Geometry: see drawing. Coordinates: mm, zero at the bounding-box minimum. A direction names the side the tool comes from. Give positions to 0.01 mm unless a question says otherwise; leave off trailing zeros. Loops run counter-clockwise (first coordinate to the right, second up) from the corner with the lowest first, then second, coordinate; pieces in that order, holes last. Notation, with made-up numbers: (30.25, -10) -> (49.25, -10) arc R33 ccw to (49.25, 18) -> close; hole circle Ø11 at (78, 16.5). An arc over 180 degrees is marked (long way). One line per question, with ' | ' between items.
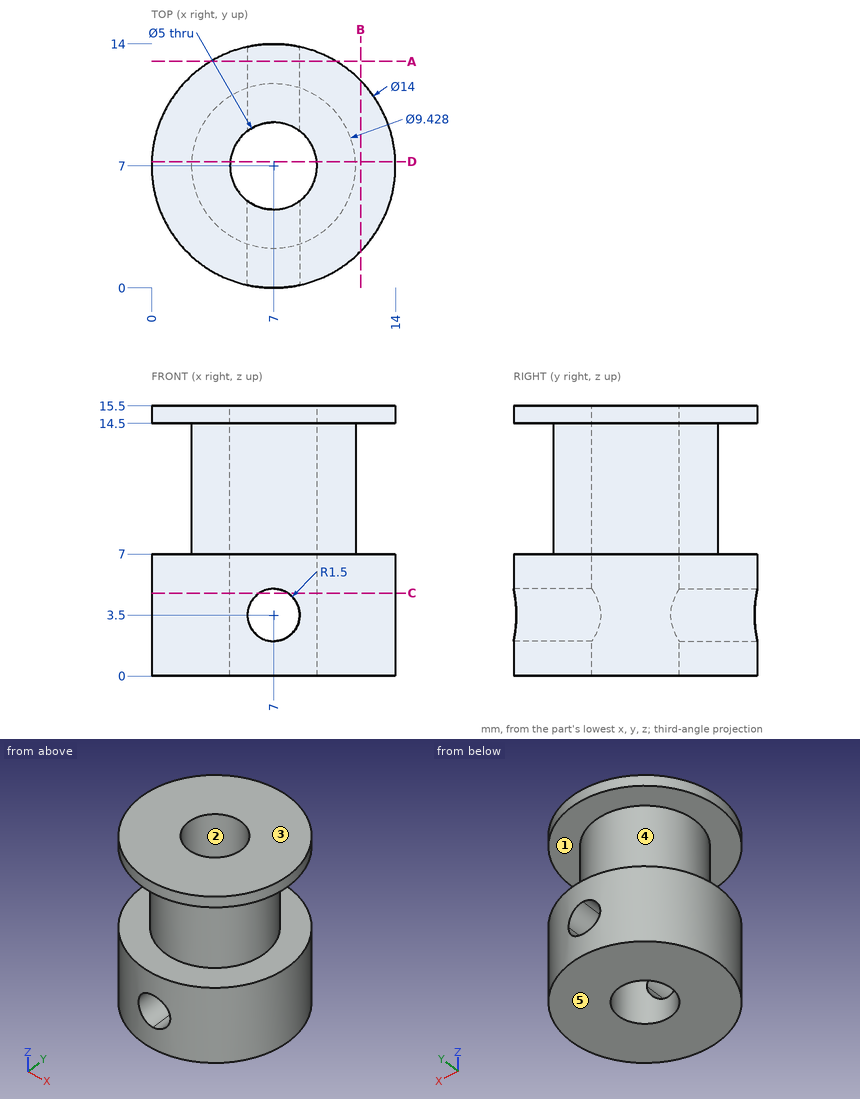
1. Reachability of the marked faces 1 and 2 from +Z, -Z, +X, -X, +Y, -Y: full face, straight path, thin tool, end or side. Return the list, or none.
Determined:
face 1: none | face 2: +Z, -Z
2. Section query D-D (y = 7.25). Output: boundary loops of the cut face in (x, z) (1 decimal).
Determined:
outline: (0, 0) -> (4.5, 0) -> (4.5, 15.5) -> (0, 15.5) -> (0, 14.5) -> (2.3, 14.5) -> (2.3, 7) -> (0, 7) -> close; (9.5, 0) -> (14, 0) -> (14, 7) -> (11.7, 7) -> (11.7, 14.5) -> (14, 14.5) -> (14, 15.5) -> (9.5, 15.5) -> close
3. Pull-direction query (Z, two-part tool) for the marked faces 3, 4 and 5; classes: pulls with the +Z half, pulls with the -Z half, needs draft (parallel to the pull), parting line crosses it, or undercut.
Determined:
face 3: pulls with the +Z half | face 4: undercut | face 5: pulls with the -Z half
4. Section query A-A (y = 13). Output: boundary loops of the cut face in (x, z) (1 decimal).
Determined:
outline: (3.4, 0) -> (10.6, 0) -> (10.6, 7) -> (3.4, 7) -> close; (3.4, 14.5) -> (10.6, 14.5) -> (10.6, 15.5) -> (3.4, 15.5) -> close; hole circle Ø3 at (7, 3.5)
5. Pin query (flat end, axial travel): P1, Ø2, axis at y = 3.5, z = 6, coming from the -X side; P2, Ø4, axis at x = 7, y = 7, coming from the +Z side; P3, Ø3, axis at y = 2.5, z = 4, coming from the -X side (1 decimal); P4, Ø2, axis at y = 2.5, z = 2.5, coming from the -X side. Return the tip coordinate at first contact, or that it passes through.
Determined:
P1: stops at x = 0.46 | P2: passes through | P3: stops at x = 0.7 | P4: stops at x = 0.94
6. Ray query, line 1 along Z through (x, y) = (10.25, 13); line 2 along X through (y, z) = (7, 9.5); line 3 along Y through (x, z) = (8.75, 13.75) (1 decimal). Return the intervals inside material, ascending. Write a range as from..to.
Determined:
line 1: z = 0..7, 14.5..15.5 | line 2: x = 2.29..4.5, 9.5..11.71 | line 3: y = 2.6..5.2, 8.8..11.4
7. Section query C-C (z = 4.75). Output: boundary loops of the cut face in (x, y), then the cut area to 3 significant figures.
Determined:
outline: (6.17, 0.05) -> (6.17, 4.64) arc R2.5 cw to (6.17, 9.36) -> (6.17, 13.95) arc R7 ccw to start; (7.83, 0.05) arc R7 ccw to (7.83, 13.95) -> (7.83, 9.36) arc R2.5 cw to (7.83, 4.64) -> close | area: 119 mm2
8. Section query B-B (x = 12). Output: boundary loops of the cut face in (y, z).
Determined:
outline: (2.1, 0) -> (11.9, 0) -> (11.9, 7) -> (2.1, 7) -> close; (2.1, 14.5) -> (11.9, 14.5) -> (11.9, 15.5) -> (2.1, 15.5) -> close
